Geometry check sheet. Reference: the model listing, model coordinates, mm. Round coordinates to 2 decimals unless told otherwise and drop trailing zeros. Order: outer loops, then holes, each group sorted by start corner. A loop starts at its lowest first (then second) coordinate and runs counter-clockwise, first axis right, second up. Notation, with made-up numbers: (70.25, 6) - (102.25, 6) arc R28 ccw to (102.25, 25) - close; hole circle Ø3 at (35, 84). An arc over 180 degrees is marked (long way). Return JSON: item names as keys, results as strings. Group by question number.
Q1. Material ranges on line 1 along Y through (x, z) = (-45.5, -0.25); line 2 along X through (y, z) = (24, -1.9); line 3 along Y through (x, z) = (-29, -0.6), recorded low to high.
Q2. Draft check along X on faces 1 (the cylindrical face through (-64.56, -31.69, -1.01)), 2 (the flat face through (-42, -3, 0)), 3 (the cylindrical face through (-36.984, 4.35, -0.986)). Enter one of: pulls with the +X half, pulls with the -X half, needs draft (parallel to the pull), parting line crosses it, or undercut.
Q3. Gauge pin test, flat end, axial feed: pin 1 Ø4 at (x, y) = (-37, 10.5) entering from +Z. Record the tip position at first contact, or that the pin passes through.
Q4. Sectioned sample at A-A, the plane z = -0.75. Record the cut outline in (x, y).
Q5. Sectioned sample at B-B, the plane x = -28. Record the cut outline in (y, z), then the cut area to 3 significant figures.
```python
from build123d import *

# Parameters (mm, degrees)
SKETCH1_W               = 40
SKETCH1_H               = 60
BOSS_EXTRUDE4_DEPTH     = 2
FILLET1_R               = 5
SKETCH12_R              = 1
CUT_EXTRUDE6_DEPTH      = 12
CUT_EXTRUDE7_DEPTH      = 8
CUT_EXTRUDE7_DEPTH_BACK = 10
SKETCH13_R              = 1
SKETCH14_R              = 1
CUT_EXTRUDE8_DEPTH      = 10


with BuildPart() as part:
    # Sketch1 → Boss-Extrude4 (new body)
    with BuildSketch(Plane.XY):
        with Locations((-45.9850693, -3.193565597)):
            Rectangle(SKETCH1_W, SKETCH1_H)
    extrude(amount=-BOSS_EXTRUDE4_DEPTH)

    # Fillet1
    fillet1_edges = [part.edges().sort_by_distance(p)[0] for p in [
        (-65.9850693, 26.806434403, -1),
        (-65.9850693, -33.193565597, -1),
        (-25.9850693, -33.193565597, -1),
        (-25.9850693, 26.806434403, -1),
    ]]
    fillet(fillet1_edges, radius=FILLET1_R)

    # Sketch12 → Cut-Extrude6 (cut)
    with BuildSketch(Plane(origin=(0, 0, -2), x_dir=(-1, 0, 0), z_dir=(0, 0, -1))):
        with Locations((45.9850693, -3.193565597)):
            Circle(SKETCH12_R)
    extrude(amount=-CUT_EXTRUDE6_DEPTH, mode=Mode.SUBTRACT)

    # Sketch13 → Cut-Extrude7 (cut, two sides: drawn at the far end of the back side and taken through both)
    with BuildSketch(Plane(origin=(0, 0, -2), x_dir=(-1, 0, 0), z_dir=(0, 0, -1)).offset(-CUT_EXTRUDE7_DEPTH_BACK)):
        with Locations((55.9850693, 4.306434403)):
            Circle(SKETCH13_R)
        with Locations((55.9850693, -10.693565597)):
            Circle(SKETCH13_R)
    extrude(amount=CUT_EXTRUDE7_DEPTH + CUT_EXTRUDE7_DEPTH_BACK, mode=Mode.SUBTRACT)

    # Sketch14 → Cut-Extrude8 (cut)
    with BuildSketch(Plane.XY):
        with Locations((-35.9850693, 4.306434403)):
            Circle(SKETCH14_R)
        with Locations((-35.9850693, -10.693565597)):
            Circle(SKETCH14_R)
    extrude(amount=-CUT_EXTRUDE8_DEPTH, mode=Mode.SUBTRACT)


solid = part.part
```
Reply:
{
 "1": {"line 1": "-33.19 to -4.07, -2.32 to 26.81", "line 2": "-65.48 to -26.49", "line 3": "-32.78 to 26.4"},
 "2": {"face 1": "pulls with the -X half", "face 2": "needs draft", "face 3": "undercut"},
 "3": {"pin 1": "z = 0"},
 "4": {"outline": "(-65.99, -28.19) arc R5 ccw to (-60.99, -33.19) - (-30.99, -33.19) arc R5 ccw to (-25.99, -28.19) - (-25.99, 21.81) arc R5 ccw to (-30.99, 26.81) - (-60.99, 26.81) arc R5 ccw to (-65.99, 21.81) - close; hole circle Ø2 at (-55.99, -10.69); hole circle Ø2 at (-55.99, 4.31); hole circle Ø2 at (-45.99, -3.19); hole circle Ø2 at (-35.99, -10.69); hole circle Ø2 at (-35.99, 4.31)"},
 "5": {"outline": "(-32.2, -2) - (25.82, -2) - (25.82, 0) - (-32.2, 0) - close", "area": "116 mm^2"}
}
